```python
from build123d import *

# Parameters (mm, degrees)
F0_W     = 660.4
F0_H     = 533.4
F1_DEPTH = 19.05
F3_R     = 12.7


# Not quite as in the source:
# - two fillets or chamfers of one size are made in one step
# - a feature of the source that left no trace in its solid (it failed there, or was rolled back) is left out


with BuildPart() as f1:
    # F0 (on Right) → F1 (new body)
    with BuildSketch(Plane.YZ):
        with Locations((-50.8608140139, 1.481294632)):
            Rectangle(F0_W, F0_H)
    extrude(amount=F1_DEPTH)

    # F3
    f3_edges = [f1.edges().sort_by_distance(p)[0] for p in [
        (9.525, -381.060814, 268.181295),
        (9.525, -381.060814, -265.218705),
        (0, -381.060814, 1.481295),
        (9.525, 279.339186, -265.218705),
        (0, -50.860814, -265.218705),
        (9.525, 279.339186, 268.181295),
        (0, 279.339186, 1.481295),
        (0, -50.860814, 268.181295),
    ]]
    fillet(f3_edges, radius=F3_R)


solid = f1.part
```
Work out the finished part from the listing and answer in its coordinate system (mm). Give positions to 0.01 mm unless a question says otherwise; leave off trailing zeros. Write each loop counter-clockwise with the first axis right and the second up, starting at its lowest first coordinate (ties: lowest second). Pieces come first, ordered by that corner, then holes. Notation, with made-up numbers: (58, 37.25) -> (71, 37.25) arc R17 cw to (71, 46.25) -> close; hole circle Ø5 at (6, 43). An arc over 180 degrees is marked (long way). Write item = value, one per line.
Q1. Flat-ended cylindrical pins translate along their axes: pin 1 Ø8 at (y, z) = (-69, 17.5) entering from -X; pin 2 Ø3 at (x, z) = (6, 27) entering from +Y; pin 3 Ø4 at (x, z) = (5, -174) entering from -Y; pin 4 Ø4 at (x, y) = (7.5, 30) entering from -Z. Find the tip coordinate at first contact, or state that the pin passes through.
Computed values:
pin_1 = 0
pin_2 = 278.23
pin_3 = -379.71
pin_4 = -264.81
Q2. Consider line 1 along Y through (x, z) = (11.25, -6.5); line 2 along Y through (x, z) = (6, -75); line 3 along Z through (x, y) = (7.5, -263). Determine where each line is inside the solid, lowest interval first.
Computed values:
line_1 = -380.98 to 279.26
line_2 = -379.15 to 277.43
line_3 = -264.11 to 267.07
Q3. Section A-A on x = 3.25 is taken. Determine the outline of the cut face in (y, z), and give its area (3 significant figures).
Computed values:
outline = (-376.85, -252.52) arc R8.48 ccw to (-368.36, -261) -> (266.64, -261) arc R8.48 ccw to (275.12, -252.52) -> (275.12, 255.48) arc R8.48 ccw to (266.64, 263.97) -> (-368.36, 263.97) arc R8.48 ccw to (-376.85, 255.48) -> close
area = 342,000 mm^2
